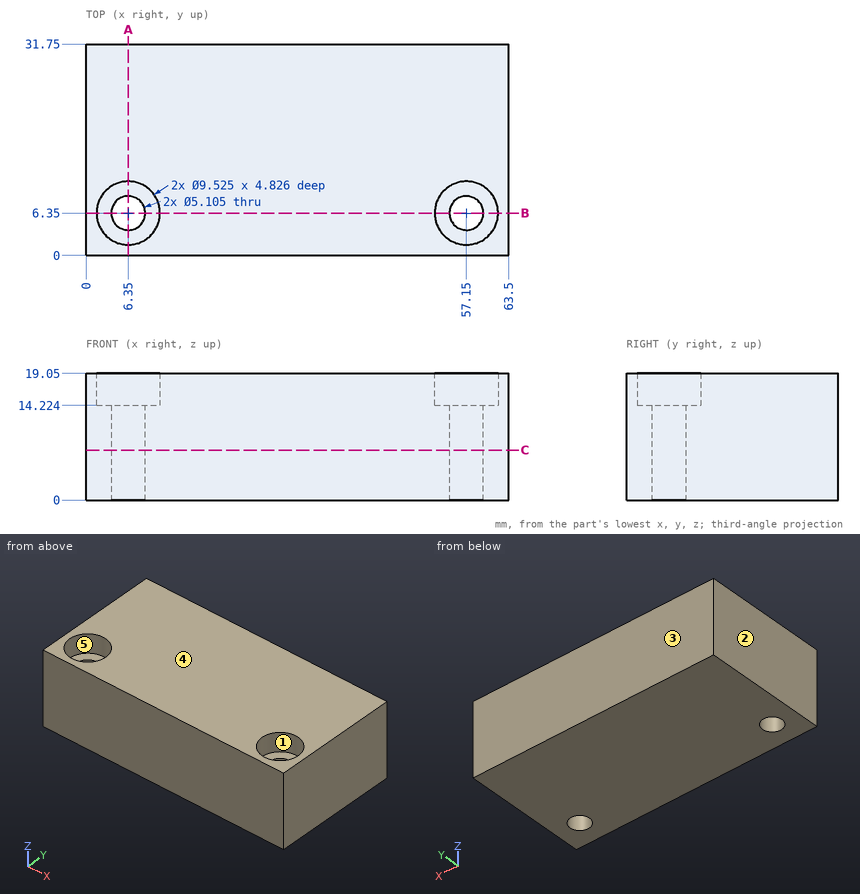
Part print with two shaded views. Sizes in mm from the minimum x, y, z corner. A direction names the side the tool comes from. Round coordinates to 2 decimals unless told otherwise and drop trailing zeros. Order: outer loops, then holes, each group sorted by start corner. A loop starts at its lowest first (then second) coordinate and runs counter-clockwise, first axis right, second up. Notation, with made-up numbers: (23.5, 35.5) - (72.5, 35.5) arc R24 cw to (72.5, 58.5) - close; hole circle Ø9 at (42, -21). An arc over 180 degrees is marked (long way). Answer as CSV lines item,"result". Start each with the question number.
1. Saw through at A-A, the plane x = 6.35. Write the cut outline in (y, z).
2. Saw through at B-B, the plane y = 6.35. Write the cut outline in (x, z).
3. Tool access for the marked faces 4 and 5: list every direction of +Z, -Z, +X, -X, +Y, -Y with a clear straight run to the whole face (end or side of a thin tool).
4. Saw through at C-C, the plane z = 7.5. Count the separate pieces of the cut face and the enclosed holes in it, and give its area (4 significant figures).
5. Pin check, flat tip, straight feed: pin 1 (5 mm diameter, centred on x = 8, y = 7, fed in from +Z). Stop position of the tip, or through.
6. Drill centre lines: L1, parallel to X at y = 6.35, z = 15.9; L2, parallel to Y at x = 6.35, z = 16.4; L3, parallel to X at y = 8, z = 5. Where is each one in solid material? Low to high. Write a range as [from, to].
7. Pull direction Y, two halves, no side cores. Call the marked faces 1, 2 and 3: +Y half, -Y half, draft (parallel to the pull), parting line (faces both ways), or undercut.
Model answer:
1,outline,"(0, 0) - (3.8, 0) - (3.8, 14.22) - (1.59, 14.22) - (1.59, 19.05) - (0, 19.05) - close; (8.9, 0) - (31.75, 0) - (31.75, 19.05) - (11.11, 19.05) - (11.11, 14.22) - (8.9, 14.22) - close"
2,outline,"(0, 0) - (3.8, 0) - (3.8, 14.22) - (1.59, 14.22) - (1.59, 19.05) - (0, 19.05) - close; (8.9, 0) - (54.6, 0) - (54.6, 14.22) - (52.39, 14.22) - (52.39, 19.05) - (11.11, 19.05) - (11.11, 14.22) - (8.9, 14.22) - close; (59.7, 0) - (63.5, 0) - (63.5, 19.05) - (61.91, 19.05) - (61.91, 14.22) - (59.7, 14.22) - close"
3,face 4,"+Z, +X, -X, +Y, -Y"
3,face 5,"+Z"
4,separate pieces,"1"
4,enclosed holes,"2"
4,area,"1,975 mm²"
5,pin 1,"stops at z = 14.22"
6,L1,"x = [0, 1.59], [11.11, 52.39], [61.91, 63.5]"
6,L2,"y = [0, 1.59], [11.11, 31.75]"
6,L3,"x = [0, 4.4], [8.3, 55.2], [59.1, 63.5]"
7,face 1,"undercut"
7,face 2,"draft"
7,face 3,"+Y half"
